from build123d import *

# Parameters (mm, degrees)
F0_W     = 50
F0_H     = 5
F1_DEPTH = 50
F2_W     = 5
F2_H     = 5.0000017802
F2_H_2   = 5
F3_DEPTH = 25
F4_R     = 4.99999


# Not quite as in the source:
# - a fillet or chamfer is up to 0.001 mm smaller than in the source, because OpenCascade refuses the exact size


with BuildPart() as f1:
    # F0 (on Front) → F1 (new body)
    with BuildSketch(Plane.XZ):
        Rectangle(F0_W, F0_H)
    extrude(amount=F1_DEPTH)

    # F2 (on face) → F3 (join)
    with BuildSketch(Plane(origin=(0, 0, -2.5), x_dir=(1, 0, 0), z_dir=(0, 0, -1))):
        with Locations((-22.5, 47.4999991099)):
            Rectangle(F2_W, F2_H)
        with Locations((22.5, 47.4999991099)):
            Rectangle(F2_W, F2_H)
        with Locations((22.5, 2.5)):
            Rectangle(F2_W, F2_H_2)
        with Locations((-22.5, 2.5)):
            Rectangle(F2_W, F2_H_2)
    extrude(amount=F3_DEPTH)

    # F4 (radius 5 in the source; OpenCascade refuses exactly that, so slightly less here)
    f4_edges = [f1.edges().sort_by_distance(p)[0] for p in [
        (-25, -50, -12.5),
        (25, -50, -12.5),
        (25, 0, -12.5),
        (-25, 0, -12.5),
    ]]
    fillet(f4_edges, radius=F4_R)


solid = f1.part
The listing builds one solid part. Answer for the finished solid, in the listing's coordinates (mm). A direction names the side the tool comes from. Coordinates: 2 decimals unless noted, no trailing zeros. Write each loop counter-clockwise with the first axis right and the second up, starting at its lowest first coordinate (ties: lowest second). Pieces come first, ordered by that corner, then holes. Notation, with made-up numbers: M 36,58.5 L 54,58.5 A21 ccw 54,64.5 Z; hole C 14.25,52 d8. An arc over 180 degrees is marked long. Put each result on its own line as item: value. Start each with the question number.
1. For a pull along X with two mould halves and no side action, classify faces 1 (the flat face through (20, -47, -15)), 2 (the cylindrical face through (-24, -2, -13)), 3 (the flat face through (25, -25, 0)), 4 (the flat face through (-23, -45, -15)) as pulls with the +X half, pulls with the -X half, needs draft (parallel to the pull), parting line crosses it, or undercut.
2. A cutting plane is placed at D-D on y = -27. Write down the section's boundary in (x, z), then the cut area to 3 significant figures.
3. A cutting plane is placed at A-A on z = -24.5. Count the separate pieces of the cut face and the enclosed holes in it, then the cut area to 3 significant figures.
4. Consider line 1 (Z direction, x = -21, y = -36.5); line 2 (Y direction, x = 21, z = -17); line 3 (Y direction, x = 21.5, z = -3). Determine where each line is inside the solid, lowest interval first. Write a range as from..to.
5. A cutting plane is placed at C-C on x = 21.5. Write down the section's boundary in (y, z), then the cut area to 3 significant figures.
6. Which of the six approach directions +Z, -Z, +X, -X, +Y, -Y give full straight-line access (tool end or side, diameter ignored) to faces 5 (the cylindrical face through (-24, -48, -12)), 6 (the flat face through (-23, -5, -15)), 7 (the flat face through (-20, -47, -15))?
7. A cutting plane is placed at B-B on y = -47. Write down the section's boundary in (x, z), then the cut area to 3 significant figures.
8. Flat-ended cylindrical pins translate along their axes: P1, Ø2, axis at x = 18.5, z = -6.5, coming from the -Y side; P2, Ø1.5, axis at y = -48, z = -16.5, coming from the +X side; P3, Ø8, axis at x = -2, y = -11, coming from the -Z side; P4, Ø1.5, axis at y = -1.5, z = -17.5, coming from the +X side. Find the tip coordinate at first contact, or state that the pin passes through.
Resolved:
1. face 1: undercut
1. face 2: pulls with the -X half
1. face 3: pulls with the +X half
1. face 4: needs draft
2. outline: M -25,-2.5 L 25,-2.5 L 25,2.5 L -25,2.5 Z
2. area: 250 mm2
3. separate pieces: 4
3. enclosed holes: 0
3. area: 78.5 mm2
4. line 1: z = -2.5..2.5
4. line 2: y = -49.9..-45, -5..-0.1
4. line 3: y = -49.77..-45, -5..-0.23
5. outline: M -49.77,-27.5 L -45,-27.5 L -45,-2.5 L -5,-2.5 L -5,-27.5 L -0.23,-27.5 L -0.23,2.5 L -49.77,2.5 Z
5. area: 486 mm2
6. face 5: +Z, -Z, -X, -Y
6. face 6: -Z, +X, -X
6. face 7: -Z, +Y, -Y
7. outline: M -24.58,-27.5 L -20,-27.5 L -20,-2.5 L 20,-2.5 L 20,-27.5 L 24.58,-27.5 L 24.58,2.5 L -24.58,2.5 Z
7. area: 475 mm2
8. P1: passes through
8. P2: stops at x = 24.47
8. P3: stops at z = -2.5
8. P4: stops at x = 24.18
